```python
from build123d import *

# Parameters (mm, degrees)
F0_R      = 9.5
F1_DEPTH  = 50
F2_R      = 25
F3_DEPTH  = 15
F5_DEPTH  = 80
F6_R      = 2.6
F7_DEPTH  = 25.001
F9_R      = 5.25
F10_DEPTH = 25
F13_DEPTH = 3.5


with BuildPart() as f1:
    # F0 (on Top) → F1 (new body)
    with BuildSketch(Plane.XY):
        Circle(F0_R)
    extrude(amount=F1_DEPTH)

    # F2 (on face) → F3 (join)
    with BuildSketch(Plane.XY.offset(50)):
        Circle(F2_R)
    extrude(amount=F3_DEPTH)

    # F4 (on face) → F5 (join)
    with BuildSketch(Plane.XY.offset(65)):
        with BuildLine():
            ThreePointArc((0, 9.5), (9.5, 0), (0, -9.5))
            Line((0, -9.5), (0, -25))
            ThreePointArc((0, -25), (17.6776695297, -17.6776695297), (25, 0))
            ThreePointArc((25, 0), (17.6776695297, 17.6776695297), (0, 25))
            Line((0, 25), (0, 9.5))
        make_face()
    extrude(amount=F5_DEPTH)

    # F6 (on face) → F7 (cut, through all)
    with BuildSketch(Plane(origin=(0, 0, 0), x_dir=(0, -1, 0), z_dir=(-1, 0, 0))):
        with Locations((17.25, 85.5)):
            Circle(F6_R)
        with Locations((17.25, 125.5)):
            Circle(F6_R)
        with Locations((-17.25, 125.5)):
            Circle(F6_R)
        with Locations((-17.25, 85.5)):
            Circle(F6_R)
    extrude(amount=-F7_DEPTH, mode=Mode.SUBTRACT)

    # F9 (on offset) → F10 (cut)
    with BuildSketch(Plane(origin=(6, 0, 0), x_dir=(0, -1, 0), z_dir=(-1, 0, 0))):
        with BuildLine():
            ThreePointArc((17.25, 120.25), (20.9623106012, 121.7876893988), (22.5, 125.5))
            ThreePointArc((22.5, 125.5), (13.5376893988, 129.2123106012), (17.25, 120.25))
        make_face()
        with Locations((-17.25, 85.5)):
            Circle(F9_R)
    extrude(amount=-F10_DEPTH, mode=Mode.SUBTRACT)

    # F12 (on offset) → F13 (cut)
    with BuildSketch(Plane.YZ.offset(-9.5)):
        with BuildLine():
            Line((-3, 33), (-3, 7))
            ThreePointArc((-3, 7), (0, 4), (3, 7))
            Line((3, 7), (3, 33))
            ThreePointArc((3, 33), (0, 36), (-3, 33))
        make_face()
    extrude(amount=F13_DEPTH, mode=Mode.SUBTRACT)


solid = f1.part
```
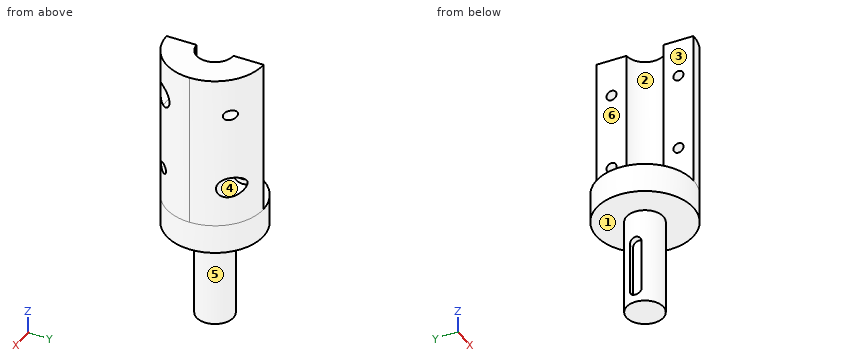
Part model, mm, in its own coordinate system. Face numbers are marked on the shaded views. A direction names the side the tool comes from. Coordinates: 2 decimals unless noted, no trailing zeros. Write each loop counter-clockwise with the first axis right and the second up, starting at its lowest first coordinate (ties: lowest second). Pieces come first, ordered by that corner, then holes.
Item 1: Slice it at D-D (y = -5.5). Write the cut outline in (x, z), and give its area (3 significant figures).
Item 2: Slice it at B-B (z = 108). Write the cut outline in (x, y).
Item 3: Which spindle directions (+Z, -Z, +X, -X, +Y, -Y) get a long thin tool onto all of the face, cutting with end or side? Do the marked faces 1, 2 and 3. Say none if no direction does.
Item 4: Slice it at C-C (y = 17.25). Write the cut outline in (x, z), and give its area (3 significant figures).
Item 5: Mould opens along Y. For the marked faces 4, 5 and 6 say: released by +Y, released by -Y, zero draft, split by the parting line, or undercut.
Item 6: Slice it at A-A (z = 85.5). Write the cut outline in (x, y), and give its area (3 significant figures).
Item 7: Pin check, flat tips, straight feed: pin 1 (12 mm diameter, centred on x = -13, y = 17.5, fed in from -Z); pin 2 (1.5 mm diameter, centred on x = -8, z = 24, fed in from +Y); pin 3 (3 mm diameter, centred on y = 17.25, z = 125.5, fed in from -X) (3 decimals); pin 4 (9.5 mm diameter, centred on y = -17.25, z = 125.5, fed in from -X). Stop position of each tip, or through.
Item 8: Probe line 1 (Z direction, x = 17.75, y = 17.25); line 2 (Z direction, x = 2, y = 17); line 3 (Z direction, x = 20, y = 3). List the from-to ranges inside material, lowest first.
Results found:
1. outline: (-24.39, 50) - (-7.75, 50) - (-7.75, 0) - (7.75, 0) - (7.75, 50) - (24.39, 50) - (24.39, 145) - (7.75, 145) - (7.75, 65) - (-24.39, 65) - close
1. area: 2,840 mm2
2. outline: (0, -25) arc R25 ccw to (0, 25) - (0, 9.5) arc R9.5 cw to (0, -9.5) - close
3. face 1: -Z
3. face 2: +Z, -X
3. face 3: +Z, -X, +Y, -Y
4. outline: (-18.1, 50) - (18.1, 50) - (18.1, 80.25) - (6, 80.25) - (6, 82.9) - (0, 82.9) - (0, 65) - (-18.1, 65) - close; (0, 88.1) - (6, 88.1) - (6, 90.75) - (18.1, 90.75) - (18.1, 122.9) - (0, 122.9) - close; (0, 128.1) - (18.1, 128.1) - (18.1, 145) - (0, 145) - close
4. area: 1,740 mm2
5. face 4: undercut
5. face 5: split by the parting line
5. face 6: zero draft
6. outline: (0, -25) arc R25 ccw to (15.2, -19.85) - (0, -19.85) - close; (0, -14.65) - (20.26, -14.65) arc R25 ccw to (21.93, 12) - (6, 12) - (6, 14.65) - (0, 14.65) - (0, 9.5) arc R9.5 cw to (0, -9.5) - close; (0, 19.85) - (6, 19.85) - (6, 22.5) - (10.9, 22.5) arc R25 ccw to (0, 25) - close
6. area: 594 mm2
7. pin 1: stops at z = 50
7. pin 2: stops at y = 6.14
7. pin 3: passes through
7. pin 4: stops at x = 0
8. line 1: z = 50 to 80.25, 90.75 to 122.9, 128.1 to 145
8. line 2: z = 50 to 82.91, 88.09 to 122.91, 128.09 to 145
8. line 3: z = 50 to 145
